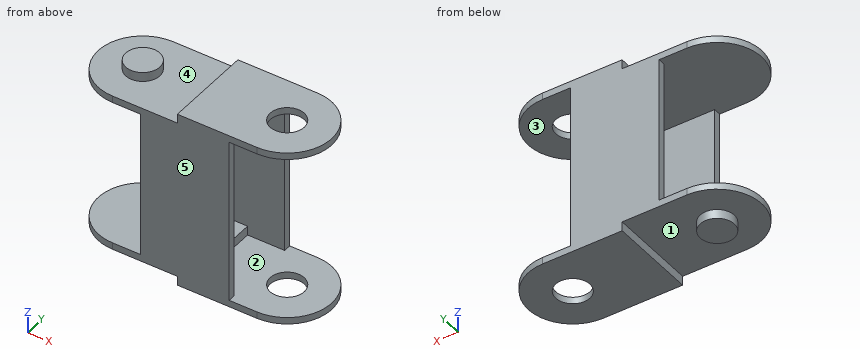
```python
from build123d import *

# Parameters (mm, degrees)
SKETCH1_R           = 2.2999954
BOSS_EXTRUDE1_DEPTH = 12.065
SKETCH2_W           = 9.75
SKETCH2_H           = 22.312
SKETCH2_W_2         = 14.75
SKETCH2_H_2         = 1.25
SKETCH2_H_3         = 19.812
CUT_EXTRUDE1_DEPTH  = 13
SKETCH3_R           = 2.2999954
BOSS_EXTRUDE2_DEPTH = 1.25
SKETCH4_R           = 2.2999954
BOSS_EXTRUDE3_DEPTH = 1.25
SKETCH5_W           = 19.812
SKETCH5_H           = 10
CUT_EXTRUDE2_DEPTH  = 22.75
SKETCH6_W           = 1.25
SKETCH6_H           = 10
CUT_EXTRUDE3_DEPTH  = 5


with BuildPart() as part:
    # Sketch1 → Boss-Extrude1 (new body, symmetric)
    with BuildSketch(Plane(origin=(0, 0, 0), x_dir=(0, 1, 0), z_dir=(0, 0, 1))):
        with BuildLine():
            Line((-6, 0), (-6, 19.5))
            ThreePointArc((-6, 19.5), (0, 25.5), (6, 19.5))
            Line((6, 19.5), (6, 0))
            ThreePointArc((6, 0), (0, -6), (-6, 0))
        make_face()
        Circle(SKETCH1_R, mode=Mode.SUBTRACT)
    extrude(amount=BOSS_EXTRUDE1_DEPTH, both=True)

    # Sketch2 → Cut-Extrude1 (cut, through all)
    with BuildSketch(Plane.XZ.offset(6)):
        with Locations((1.125, 0)):
            Rectangle(SKETCH2_W, SKETCH2_H)
        with Locations((-18.125, 11.44)):
            Rectangle(SKETCH2_W_2, SKETCH2_H_2)
        with Locations((-18.125, -11.44)):
            Rectangle(SKETCH2_W_2, SKETCH2_H_2)
        with Locations((-20.625, 0)):
            Rectangle(SKETCH2_W, SKETCH2_H_3)
    extrude(amount=-CUT_EXTRUDE1_DEPTH, mode=Mode.SUBTRACT)

    # Sketch3 → Boss-Extrude2 (add)
    with BuildSketch(Plane.XY.offset(10.815)):
        with Locations((-19.5, 0)):
            Circle(SKETCH3_R)
    extrude(amount=BOSS_EXTRUDE2_DEPTH)

    # Sketch4 → Boss-Extrude3 (add)
    with BuildSketch(Plane(origin=(0, 0, -10.815), x_dir=(1, 0, 0), z_dir=(0, 0, -1))):
        with Locations((-19.5, 0)):
            Circle(SKETCH4_R)
    extrude(amount=BOSS_EXTRUDE3_DEPTH)

    # Sketch5 → Cut-Extrude2 (cut, through all)
    with BuildSketch(Plane(origin=(-3.75, 0, 0), x_dir=(0, 0, -1), z_dir=(1, 0, 0))):
        Rectangle(SKETCH5_W, SKETCH5_H)
    extrude(amount=-CUT_EXTRUDE2_DEPTH, mode=Mode.SUBTRACT)

    # Sketch6 → Cut-Extrude3 (cut)
    with BuildSketch(Plane(origin=(-3.75, 0, 0), x_dir=(0, 0, -1), z_dir=(1, 0, 0))):
        with Locations((-10.531, 0)):
            Rectangle(SKETCH6_W, SKETCH6_H)
        with Locations((10.531, 0)):
            Rectangle(SKETCH6_W, SKETCH6_H)
    extrude(amount=-CUT_EXTRUDE3_DEPTH, mode=Mode.SUBTRACT)


solid = part.part
```
Work out the finished part from the listing and answer in its coordinate system (mm). Face numbers are marked on the shaded views. A direction names the side the tool comes from. Give positions to 0.01 mm unless a question says otherwise; leave off trailing zeros. Loops run counter-clockwise (first coordinate to the right, second up) from the corner with the lowest first, then second, coordinate; pieces in that order, holes last. Notation, with made-up numbers: (70.5, 60) - (99.5, 60) arc R12 ccw to (99.5, 82) - close; hole circle Ø7 at (-16.75, 65.5). An arc over 180 degrees is marked (long way). Use CSV: the item, a comma, the result in double quotes. Start each with the question number.
(1) Find section D-D, the plane y = -3.5. Determine the outline of the cut face in (x, z) (3 decimals), plus the area to 3 significant figures.
(2) Find section A-A, the plane x = -3. Determine the outline of the cut face in (y, z) (3 decimals), plus the area to 3 significant figures.
(3) Determine the mould class of the marked faces 1 and 2 for opening direction X: released by +X, released by -X, zero draft, split by the parting line, or undercut.
(4) Find section B-B, the plane z = 3.75. Determine the outline of the cut face in (x, y), plus the area to 3 significant figures.
(5) A tool of negligible diameter and unlimited length cuts with its end or side. For the marked faces 3, 4 and 5, from which of +Z, -Z, +X, -X, +Y, -Y can it reach the whole face along a straight path? Write none if from no direction.
(6) Find section C-C, the plane y = 0. Count the separate pieces of the cut face and the enclosed holes in it, plus the area to 3 significant figures.
(7) Find the intervals of material crossed by L1, parallel to X at y = 0, z = -11.5; L2, parallel to Z at x = -1, y = 5.75 (3 decimals); L3, parallel to Z at x = -11.5, y = 0 (3 decimals), in increasing order.
(8) Each of these flat-tipped pins is pushed along its axis until it touches: pin 1 (1 mm diameter, centred on y = -3, z = 6, fed in from +X); pin 2 (0.6 mm diameter, centred on y = -0.5, z = -10.5, fed in from +X); pin 3 (0.5 mm diameter, centred on y = -5.5, z = -0.5, fed in from +X); pin 4 (0.8 mm diameter, centred on y = 5.5, z = 0.5, fed in from -X). Where does it stop, or does it pass through?
Results found:
1,outline,"(-24.373, -10.815) - (-10.75, -10.815) - (-10.75, -12.065) - (4.873, -12.065) - (4.873, -11.156) - (-8.75, -11.156) - (-8.75, -9.906) - (-24.373, -9.906) - close; (-24.373, 9.906) - (-8.75, 9.906) - (-8.75, 11.156) - (4.873, 11.156) - (4.873, 12.065) - (-10.75, 12.065) - (-10.75, 10.815) - (-24.373, 10.815) - close"
1,area,"58.2 mm^2"
2,outline,"(-6, -12.065) - (6, -12.065) - (6, -11.156) - (-6, -11.156) - close; (-6, 11.156) - (6, 11.156) - (6, 12.065) - (-6, 12.065) - close"
2,area,"21.8 mm^2"
3,face 1,"undercut"
3,face 2,"zero draft"
4,outline,"(-15.75, -6) - (-3.75, -6) - (-3.75, -5) - (-15.75, -5) - close; (-15.75, 5) - (-3.75, 5) - (-3.75, 6) - (-15.75, 6) - close"
4,area,"24.0 mm^2"
5,face 3,"+X"
5,face 4,"+Z"
5,face 5,"+Z, -Z, +X, -X, -Y"
6,separate pieces,"4"
6,enclosed holes,"0"
6,area,"65.4 mm^2"
7,L1,"-21.8 to -17.2, -10.75 to -2.3, 2.3 to 6"
7,L2,"-12.065 to -11.156, 11.156 to 12.065"
7,L3,"-10.815 to -9.906, 9.906 to 10.815"
8,pin 1,"through"
8,pin 2,"x = -8.75"
8,pin 3,"x = -3.75"
8,pin 4,"x = -15.75"
